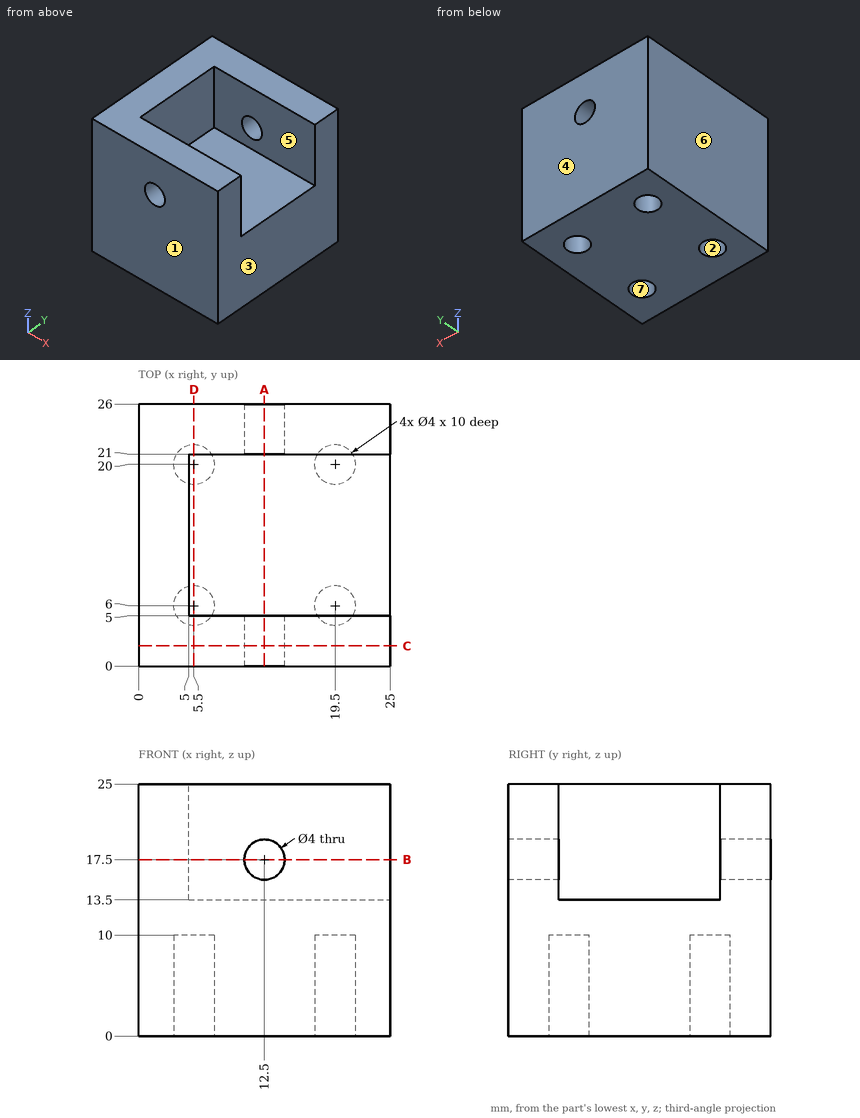
Geometry check sheet. Reference: drawing and pictorial views, mm from the part's lowest x, y, z. A direction names the side the tool comes from. Coordinates: 2 decimals unless noted, no trailing zeros. Order: outer loops, then holes, each group sorted by start corner. A loop starts at its lowest first (then second) coordinate and runs counter-clockwise, first axis right, second up. Notation, with made-up numbers: (-38.75, 78.5) - (-15.75, 78.5) arc R27 ccw to (-15.75, 104.5) - close; hole circle Ø4 at (84, 45). An arc over 180 degrees is marked (long way). Answer in a Markdown table with one row per item. Add a question column.
1) Material ranges on line 1 along X through (y, z) = (6, 7); line 2 along Z through (x, y) = (12.5, 1.05); line 3 along Y through (x, z) = (5, 4.75), recorded low to high. Write a range as [from, to].
2) Cross-section at D-D, the plane x = 5.5. Record the cut outline in (y, z).
3) Cross-section at B-B, the plane z = 17.5. Record the cut outline in (x, y), then the cut area to 3 significant figures.
4) Cross-section at C-C, the plane y = 2. Record the cut outline in (x, z), then the cut area to 3 significant figures.
5) Cross-section at A-A, the plane x = 12.5. Record the cut outline in (y, z), then the cut area to 3 significant figures.
6) Gauge pin test, flat ends, axial feed: P1, Ø13, axis at x = 17.5, y = 13.5, coming from the +Z side; P2, Ø8, axis at y = 16.5, z = 18, coming from the +X side. Record the tip position at first contact, or that the pin passes through.
7) Release check for a two-part mould opening along Y. For the marked faces 1, 2, 3 and 4 record: +Y half, -Y half, draft (parallel to the pull), parting line (faces both ways), or undercut.
8) Set-up check for the marked faces 5, 6 and 7: record each of +Z, -Z, +X, -X, +Y, -Y from which the full face is reachable in a straight line by a thin tool's end or side.
Check result:
| question | item | result |
|---|---|---|
| 1 | line 1 | x = [0, 3.5], [7.5, 17.5], [21.5, 25] |
| 1 | line 2 | z = [0, 15.5], [19.5, 25] |
| 1 | line 3 | y = [0, 4.06], [7.94, 18.06], [21.94, 26] |
| 2 | outline | (0, 0) - (4, 0) - (4, 10) - (8, 10) - (8, 0) - (18, 0) - (18, 10) - (22, 10) - (22, 0) - (26, 0) - (26, 25) - (21, 25) - (21, 13.5) - (5, 13.5) - (5, 25) - (0, 25) - close |
| 3 | outline | (0, 0) - (10.5, 0) - (10.5, 5) - (5, 5) - (5, 21) - (10.5, 21) - (10.5, 26) - (0, 26) - close; (14.5, 0) - (25, 0) - (25, 5) - (14.5, 5) - close; (14.5, 21) - (25, 21) - (25, 26) - (14.5, 26) - close |
| 3 | area | 290 mm² |
| 4 | outline | (0, 0) - (25, 0) - (25, 25) - (0, 25) - close; hole circle Ø4 at (12.5, 17.5) |
| 4 | area | 612 mm² |
| 5 | outline | (0, 0) - (26, 0) - (26, 15.5) - (21, 15.5) - (21, 13.5) - (5, 13.5) - (5, 15.5) - (0, 15.5) - close; (0, 19.5) - (5, 19.5) - (5, 25) - (0, 25) - close; (21, 19.5) - (26, 19.5) - (26, 25) - (21, 25) - close |
| 5 | area | 426 mm² |
| 6 | P1 | stops at z = 13.5 |
| 6 | P2 | stops at x = 5 |
| 7 | face 1 | -Y half |
| 7 | face 2 | undercut |
| 7 | face 3 | draft |
| 7 | face 4 | +Y half |
| 8 | face 5 | +Z, +X |
| 8 | face 6 | +Z, -Z, -X, +Y, -Y |
| 8 | face 7 | -Z |
